Input: part model. Units: mm. Frame: model coordinates. Face numbers are marked on the shaded views. A direction names the side the tool comes from. Give positions to 0.01 mm unless a question says otherwise; leave off trailing zeros. Loops run counter-clockwise (first coordinate to the right, second up) from the corner with the lowest first, then second, coordinate; pieces in that order, holes last. Notation, with made-up numbers: (4, 80) - (25, 80) arc R37 ccw to (25, 117) - close; hole circle Ø5 at (52.5, 10.5). An arc over 180 degrees is marked (long way). Answer as a JSON object with one key per item and string values.
from build123d import *

# Parameters (mm, degrees)
ESBO_O1_W                = 28
ESBO_O1_H                = 38
RESSALTO_EXTRUS_O1_DEPTH = 5.5
ESBO_O2_W                = 28
ESBO_O2_H                = 5.5
RESSALTO_EXTRUS_O2_DEPTH = 32.5
CORTE_EXTRUS_O1_DEPTH    = 28
RESSALTO_EXTRUS_O3_DEPTH = 28
CORTE_EXTRUS_O2_DEPTH    = 0.15
CORTE_EXTRUS_O3_DEPTH    = 0.15
ESBO_O8_R                = 3
CORTE_EXTRUS_O4_DEPTH    = 6
ESBO_O9_R                = 3
CORTE_EXTRUS_O5_DEPTH    = 6


with BuildPart() as part:
    # Esboço1 → Ressalto-extrusão1 (new body)
    with BuildSketch(Plane.XY):
        with Locations((-17.133729377, 2.988196373)):
            Rectangle(ESBO_O1_W, ESBO_O1_H)
    extrude(amount=RESSALTO_EXTRUS_O1_DEPTH)

    # Esboço2 → Ressalto-extrusão2 (add)
    with BuildSketch(Plane.XY.offset(5.5)):
        with Locations((-17.133729377, -13.261803627)):
            Rectangle(ESBO_O2_W, ESBO_O2_H)
    extrude(amount=RESSALTO_EXTRUS_O2_DEPTH)

    # Esboço3 → Corte-extrusão1 (cut)
    with BuildSketch(Plane.ZY.offset(31.133729377)):
        with BuildLine():
            Line((1.5, 21.988196373), (5.5, 21.988196373))
            Line((5.5, 21.988196373), (5.5, 17.988196373))
            ThreePointArc((5.5, 17.988196373), (4.328427125, 20.816623498), (1.5, 21.988196373))
        make_face()
        with BuildLine():
            Line((34, -10.511803627), (38, -10.511803627))
            Line((38, -10.511803627), (38, -14.511803627))
            ThreePointArc((38, -14.511803627), (36.828427125, -11.683376502), (34, -10.511803627))
        make_face()
    extrude(amount=-CORTE_EXTRUS_O1_DEPTH, mode=Mode.SUBTRACT)

    # Esboço4 → Ressalto-extrusão3 (add)
    with BuildSketch(Plane.ZY.offset(31.133729377)):
        Polygon((5.5, -10.511803627), (12.1, -10.511803627), (5.5, -3.911803627), align=None)
    extrude(amount=-RESSALTO_EXTRUS_O3_DEPTH)

    # Esboço5 → Corte-extrusão2 (cut)
    with BuildSketch(Plane.XZ.offset(16.011803627)):
        Polygon((-25.633729377, 5.5), (-25.633729377, 0), (-8.633729377, 0), (-8.633729377, 5.5), (-3.133729377, 5.5), (-3.133729377, 32.5), (-8.633729377, 32.5), (-8.633729377, 38), (-25.633729377, 38), (-25.633729377, 32.5), (-31.133729377, 32.5), (-31.133729377, 5.5), align=None)
    extrude(amount=-CORTE_EXTRUS_O2_DEPTH, mode=Mode.SUBTRACT)

    # Esboço6 → Corte-extrusão3 (cut)
    with BuildSketch(Plane(origin=(0, 0, 0), x_dir=(-1, 0, 0), z_dir=(0, 0, -1))):
        Polygon((8.633729377, -10.511803627), (8.633729377, -15.861803627), (25.633729377, -15.861803627), (25.633729377, -10.511803627), (31.133729377, -10.511803627), (31.133729377, 16.488196373), (25.633729377, 16.488196373), (25.633729377, 21.988196373), (8.633729377, 21.988196373), (8.633729377, 16.488196373), (3.133729377, 16.488196373), (3.133729377, -10.511803627), align=None)
    extrude(amount=-CORTE_EXTRUS_O3_DEPTH, mode=Mode.SUBTRACT)

    # Esboço8 → Corte-extrusão4 (cut)
    with BuildSketch(Plane.XZ.offset(15.861803627)):
        with Locations(Location((-17.133729377, 26, 0), (0, 0, 270))):
            Circle(ESBO_O8_R)
    extrude(amount=-CORTE_EXTRUS_O4_DEPTH, mode=Mode.SUBTRACT)

    # Esboço9 → Corte-extrusão5 (cut)
    with BuildSketch(Plane(origin=(0, 0, 0.15), x_dir=(-1, 0, 0), z_dir=(0, 0, -1))):
        with Locations((17.133729377, 9.988196373)):
            Circle(ESBO_O9_R)
    extrude(amount=-CORTE_EXTRUS_O5_DEPTH, mode=Mode.SUBTRACT)


solid = part.part
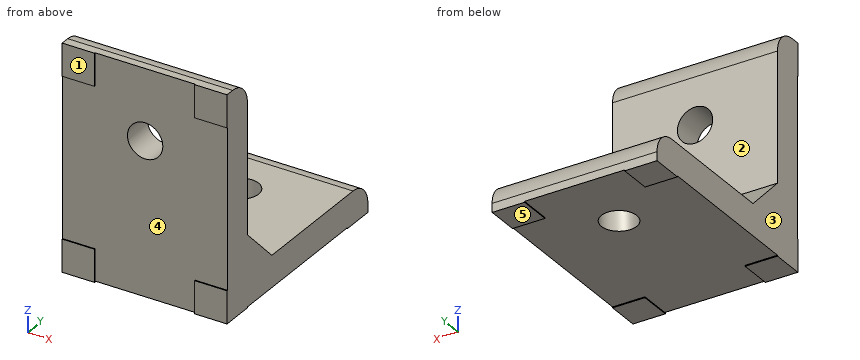
Item 1: Contact query for flat-ended pins moving along their axis: P1, Ø10, axis at x = -9, y = 6.5, coming from the -Z side; P2, Ø5, axis at x = -15.5, z = 26.5, coming from the +Y side; P3, Ø2, axis at x = -18, z = 4, coming from the +Y side. Output: stop coordinate, or through.
Geometry check:
{"P1": "stops at z = 0.15", "P2": "stops at y = -10.51", "P3": "stops at y = 21.7"}
Item 2: Material intervals for line 1 (X direction, y = -11.8, z = 26); line 2 (Y direction, x = -10, z = 30); line 3 (Z direction, x = -29, y = 0), sorted ascending. Write a range as [from, to].
Geometry check:
{"line 1": "x = [-31.13, -20.13], [-14.13, -3.13]", "line 2": "y = [-15.86, -10.51]", "line 3": "z = [0.15, 5.5]"}
Item 3: Access query for the marked faces 1 and 2. Directions: +Z, -Z, +X, -X, +Y, -Y. A direction counts if a zero-diameter tool reaches every point of the face in a straight line with its end or side. Return the directions, or none.
Geometry check:
{"face 1": "+Z, -Z, +X, -X, -Y", "face 2": "+Z, +X, -X, +Y"}
Item 4: Cut plane A-A (z = 26). Return loops of the section in (x, y).
Geometry check:
{"outline": "(-31.13, -15.86) - (-20.13, -15.86) - (-20.13, -10.51) - (-31.13, -10.51) - close; (-14.13, -15.86) - (-3.13, -15.86) - (-3.13, -10.51) - (-14.13, -10.51) - close"}
Item 5: Cut plane D-D (x = -9.75). Return loops of the section in (y, z).
Geometry check:
{"outline": "(-15.86, 0.15) - (21.99, 0.15) - (21.99, 1.5) arc R4 ccw to (17.99, 5.5) - (-3.91, 5.5) - (-10.51, 12.1) - (-10.51, 34) arc R4 ccw to (-14.51, 38) - (-15.86, 38) - close"}
Item 6: Cut plane C-C (y = 9). Return loops of the section in (x, z).
Geometry check:
{"outline": "(-31.13, 0.15) - (-19.97, 0.15) - (-19.97, 5.5) - (-31.13, 5.5) - close; (-14.3, 0.15) - (-3.13, 0.15) - (-3.13, 5.5) - (-14.3, 5.5) - close"}
Item 7: Cut plane B-B (x = -27). Return loops of the section in (y, z).
Geometry check:
{"outline": "(-16.01, 0) - (-10.51, 0) - (-10.51, 0.15) - (16.49, 0.15) - (16.49, 0) - (21.99, 0) - (21.99, 1.5) arc R4 ccw to (17.99, 5.5) - (-3.91, 5.5) - (-10.51, 12.1) - (-10.51, 34) arc R4 ccw to (-14.51, 38) - (-16.01, 38) - (-16.01, 32.5) - (-15.86, 32.5) - (-15.86, 5.5) - (-16.01, 5.5) - close"}
Item 8: Mould query, pull axis X, two halves, no side actions, for the marked faces 3, 4 and 5. Classes: released by +X, released by -X, zero draft, split by the parting line, or undercut.
Geometry check:
{"face 3": "released by -X", "face 4": "undercut", "face 5": "zero draft"}
